```python
from build123d import *

# Parameters (mm, degrees)
SKETCH1_W           = 129.286
SKETCH1_H           = 16.51
BOSS_EXTRUDE1_DEPTH = 3.175
FILLET1_R           = 8.128
SKETCH2_R           = 1.4605
CUT_EXTRUDE1_DEPTH  = 66.24525346


with BuildPart() as part:
    # Sketch1 → Boss-Extrude1 (new body)
    with BuildSketch(Plane.XY):
        Rectangle(SKETCH1_W, SKETCH1_H)
    extrude(amount=BOSS_EXTRUDE1_DEPTH)

    # Fillet1
    fillet1_edges = [part.edges().sort_by_distance(p)[0] for p in [
        (64.643, -8.255, 1.5875),
        (-64.643, -8.255, 1.5875),
        (-64.643, 8.255, 1.5875),
        (64.643, 8.255, 1.5875),
    ]]
    fillet(fillet1_edges, radius=FILLET1_R)

    # Sketch2 → Cut-Extrude1 (cut, through all)
    with BuildSketch(Plane.XY.offset(3.175)):
        with Locations((-56.515, 0.127)):
            Circle(SKETCH2_R)
        with Locations((56.515, -0.127)):
            Circle(SKETCH2_R)
    extrude(amount=-CUT_EXTRUDE1_DEPTH, mode=Mode.SUBTRACT)


solid = part.part
```
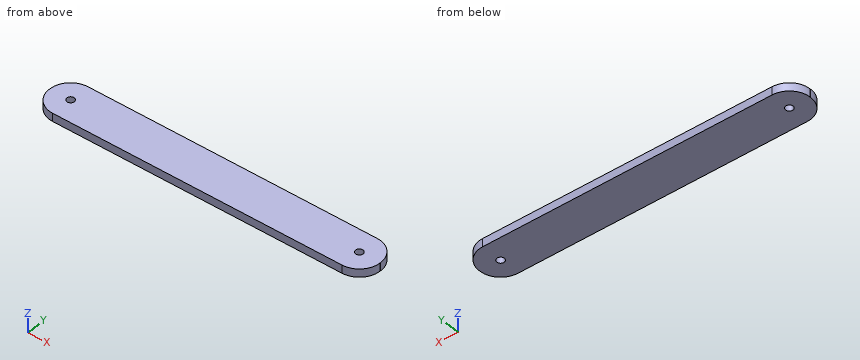
Part model, mm, in its own coordinate system. Coordinates: 2 decimals unless noted, no trailing zeros. Write each loop counter-clockwise with the first axis right and the second up, starting at its lowest first coordinate (ties: lowest second). Pieces come first, ordered by that corner, then holes.
Item 1: Slice it at C-C (y = -5.75). Write the cut outline in (x, z) (3 decimals).
Item 2: Slice it at B-B (y = 5.25). Write the cut outline in (x, z) (3 decimals).
Item 3: Probe line 1 (X direction, y = 4.25, z = 1); line 2 (X direction, y = -4.75, z = 0.8). List the from-to ranges inside material, lowest first.
Item 4: Slice it at A-A (z = 1.75). Count the separate pieces of the cut face and the enclosed holes in it, and give its area (3 significant figures).
Results found:
1. outline: (-62.384, 0) - (62.384, 0) - (62.384, 3.175) - (-62.384, 3.175) - close
2. outline: (-62.825, 0) - (62.825, 0) - (62.825, 3.175) - (-62.825, 3.175) - close
3. line 1: x = -63.52 to 63.52
3. line 2: x = -63.2 to 63.2
4. separate pieces: 1
4. enclosed holes: 2
4. area: 2,060 mm2
